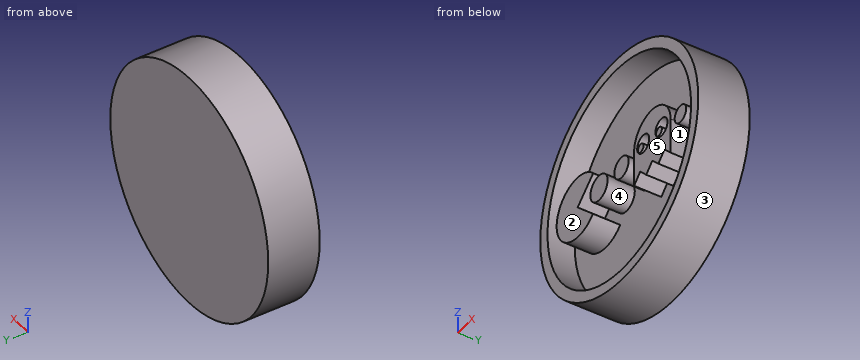
```python
from build123d import *

# Parameters (mm, degrees)
F0_R     = 27.5
F1_DEPTH = 12
F2_R     = 25
F3_DEPTH = 6.35
F4_R     = 3
F4_R_2   = 2.1
F4_R_3   = 2.5
F4_R_4   = 2
F4_R_5   = 1
F5_DEPTH = 6.35


with BuildPart() as f1:
    # F0 (on Front) → F1 (new body)
    with BuildSketch(Plane.XZ):
        Circle(F0_R)
    extrude(amount=F1_DEPTH)

    # F2 (on face) → F3 (cut)
    with BuildSketch(Plane.XZ.offset(12)):
        Circle(F2_R)
    extrude(amount=-F3_DEPTH, mode=Mode.SUBTRACT)

    # F4 (on face) → F5 (join)
    with BuildSketch(Plane.XZ.offset(5.65)):
        with BuildLine():
            Line((-14.503664, 0), (-9.082651, 4.892762))
            ThreePointArc((-9.082651, 4.892762), (-21.805957, 0.055061), (-9.157048, -4.973953))
            Line((-9.157048, -4.973953), (-14.503664, 0))
        make_face()
        with Locations((-7.077939, 0)):
            Circle(F4_R)
        with BuildLine():
            ThreePointArc((17.865209, 0.9525), (11.515209, 7.3025), (5.165209, 0.9525))
            Line((5.165209, 0.9525), (5.165209, -7.3025))
            Line((5.165209, -7.3025), (7.281875, -5.185833))
            Line((7.281875, -5.185833), (9.398542, -7.3025))
            Line((9.398542, -7.3025), (11.515209, -5.185833))
            Line((11.515209, -5.185833), (13.631875, -7.3025))
            Line((13.631875, -7.3025), (15.748542, -5.185833))
            Line((15.748542, -5.185833), (17.865209, -7.3025))
            Line((17.865209, -7.3025), (17.865209, 0.9525))
        make_face()
        with Locations((8.340209, 0.9525)):
            Circle(F4_R_2, mode=Mode.SUBTRACT)
        with Locations((14.690209, 0.9525)):
            Circle(F4_R_2, mode=Mode.SUBTRACT)
        with Locations((0.767446, 0)):
            Circle(F4_R_3)
        with Locations((21.29638, 0)):
            Circle(F4_R_4)
        with Locations((7.478851, 0.4445)):
            Circle(F4_R_5)
        with Locations((13.828851, 0.4445)):
            Circle(F4_R_5)
    extrude(amount=F5_DEPTH)


solid = f1.part
```
Read the model definition and answer for the solid it produces. Units are mm, in the model's axes. Face numbers are marked on the shaded views. A direction names the side the tool comes from. Coordinates: 2 decimals unless noted, no trailing zeros. Write each loop counter-clockwise with the first axis right and the second up, starting at its lowest first coordinate (ties: lowest second). Pieces come first, ordered by that corner, then holes. Notation, with made-up numbers: (-31.5, 51.25) -> (-6.5, 51.25) arc R10 ccw to (-6.5, 63.25) -> close; hole circle Ø3 at (75, -24.5). An arc over 180 degrees is marked (long way). Answer as a JSON object with one key per item and string values.
Q1. Flat-ended cylindrical pins translate along their axes: pin 1 Ø3 at (y, z) = (-10, -4.5) entering from -X; pin 2 Ø2 at (x, y) = (14.5, -6) entering from -Z; pin 3 Ø2 at (x, y) = (0.5, -2.5) entering from +Z. Find the tip coordinate at first contact, or state that the pin passes through.
The answers:
{"pin 1": "stops at x = -27.34", "pin 2": "stops at z = -23.96", "pin 3": "stops at z = 27.5"}
Q2. The part is cut by section A-A on y = -7. Give the number of separate pieces and of enclosed holes in the cut face, then the cut area to 3 significant figures.
The answers:
{"separate pieces": "8", "enclosed holes": "3", "area": "734 mm2"}
Q3. A tool of negligible diameter and unlimited length cuts with its end or side. For the marked faces 4 and 5, from which of +Z, -Z, +X, -X, +Y, -Y can it reach the whole face along a straight path? Write none if from no direction.
The answers:
{"face 4": "-Y", "face 5": "+Z, -Z, +X, -X, -Y"}
Q4. The part is cut by section B-B on x = 0. Give the vertices of the cut face in (y, z), then the cut area to 3 significant figures.
The answers:
{"outline": "(-12, -27.5) -> (0, -27.5) -> (0, 27.5) -> (-12, 27.5) -> (-12, 25) -> (-5.65, 25) -> (-5.65, 2.38) -> (-12, 2.38) -> (-12, -2.38) -> (-5.65, -2.38) -> (-5.65, -25) -> (-12, -25) -> close", "area": "373 mm2"}
Q5. The part is cut by section D-D on y = -3.25. Give the vertices of the cut face in (x, z), then the cut area to 3 significant figures.
The answers:
{"outline": "circle Ø55 at (0, 0)", "area": "2,380 mm2"}
Q6. Determine the mould class of the marked faces 1, 2 and 3 for opening direction X: pulls with the +X half, pulls with the -X half, needs draft (parallel to the pull), parting line crosses it, or undercut.
The answers:
{"face 1": "undercut", "face 2": "needs draft", "face 3": "parting line crosses it"}
Q7. Consider line 1 (Z direction, x = 0, y = -8.25); line 2 (Y direction, x = 4.5, z = -19); line 3 (Z direction, x = -11, y = -7). Determine where each line is inside the solid, lowest interval first. Write a range as [from, to].
The answers:
{"line 1": "z = [-27.5, -25], [-2.38, 2.38], [25, 27.5]", "line 2": "y = [-5.65, 0]", "line 3": "z = [-25.2, -22.45], [-6.41, -3.26], [3.16, 6.41], [22.45, 25.2]"}
Q8. The part is cut by section C-C on z = -10. Give the vertices of the cut face in (x, y), then the cut area to 3 significant figures.
The answers:
{"outline": "(-25.62, -12) -> (-22.91, -12) -> (-22.91, -5.65) -> (22.91, -5.65) -> (22.91, -12) -> (25.62, -12) -> (25.62, 0) -> (-25.62, 0) -> close", "area": "324 mm2"}
